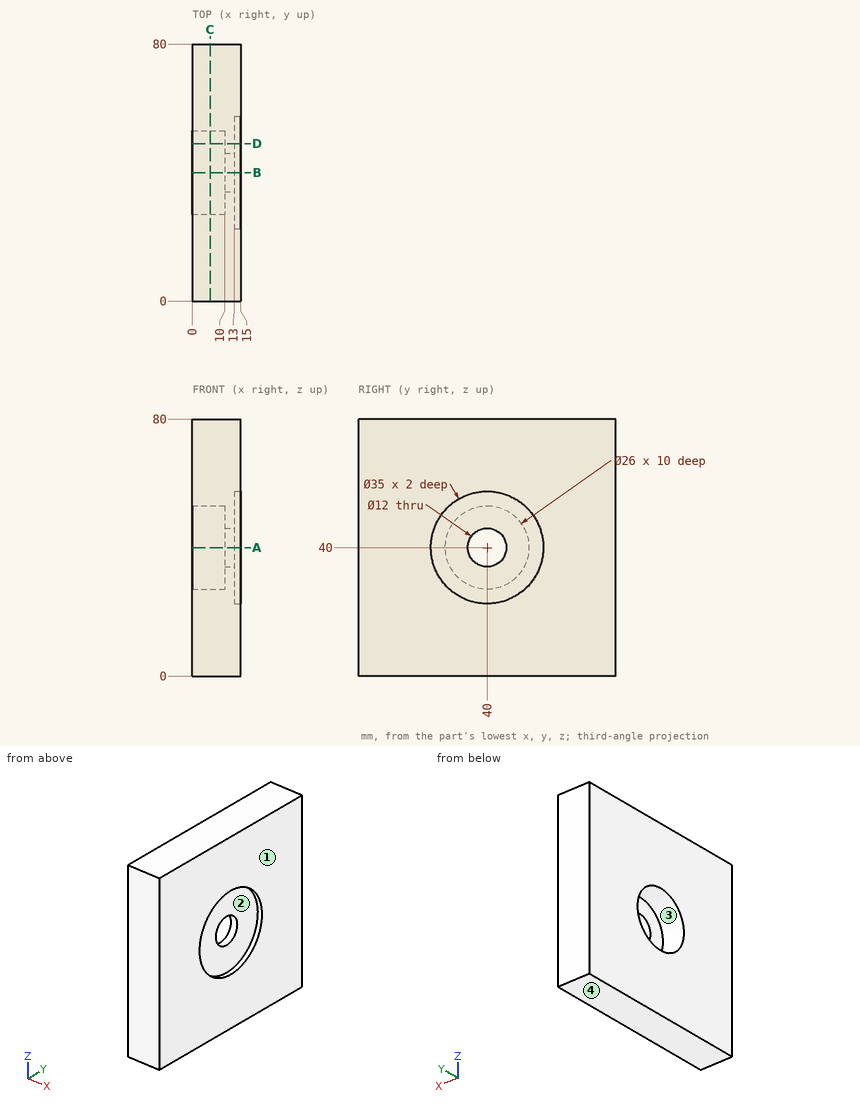
Check sheet for the drawn part. Datum: minimum x, y, z corner. Units: mm. Round coordinates to 2 decimals unless told otherwise and drop trailing zeros. Order: outer loops, then holes, each group sorted by start corner. A loop starts at its lowest first (then second) coordinate and runs counter-clockwise, first axis right, second up. Notation, with made-up numbers: M 17,69 L 26,69 A25 cw 26,100 Z; hole C -17,-21 d8. An arc over 180 degrees is marked long. Answer in a Markdown table with one row per item.
(1) Section check C-C on x = 5.5. Record the boundary of the cut face in (y, z).
Findings:
| item | result |
|---|---|
| outline | M 0,0 L 80,0 L 80,80 L 0,80 Z; hole C 40,40 d26 |
(2) Section check A-A on z = 40. Record the boundary of the cut face in (x, y), plus the area to 3 significant figures.
Findings:
| item | result |
|---|---|
| outline | M 0,0 L 15,0 L 15,22.5 L 13,22.5 L 13,34 L 10,34 L 10,27 L 0,27 Z; M 0,53 L 10,53 L 10,46 L 13,46 L 13,57.5 L 15,57.5 L 15,80 L 0,80 Z |
| area | 834 mm^2 |
(3) Section check D-D on y = 49. Record the boundary of the cut face in (x, z), plus the area to 3 significant figures.
Findings:
| item | result |
|---|---|
| outline | M 0,0 L 15,0 L 15,24.99 L 13,24.99 L 13,55.01 L 15,55.01 L 15,80 L 0,80 L 0,49.38 L 10,49.38 L 10,30.62 L 0,30.62 Z |
| area | 952 mm^2 |
(4) Gauge pin test, flat ends, axial feed: pin 1 (11 mm diameter, centred on y = 40, z = 40, fed in from +X); pin 2 (6 mm diameter, centred on x = 7, y = 68.5, fed in from -Z); pin 3 (17.5 mm diameter, centred on y = 47, z = 36, fed in from +X); pin 4 (8 mm diameter, centred on y = 43.5, z = 43.5, fed in from -X). Record the tip position at first contact, or that the pin passes through.
Findings:
| item | result |
|---|---|
| pin 1 | passes through |
| pin 2 | stops at z = 0 |
| pin 3 | stops at x = 13 |
| pin 4 | stops at x = 10 |
(5) Draft check along Z on the marked faces 1, 2, 3 and 4. Enter one of: +Z half, -Z half, draft (parallel to the pull), parting line (faces both ways), or undercut.
Findings:
| item | result |
|---|---|
| face 1 | draft |
| face 2 | undercut |
| face 3 | undercut |
| face 4 | -Z half |
(6) Material ranges on line 1 along Y through (x, z) = (4, 40); line 2 along Y through (x, z) = (11.7, 40); line 3 along Z through (x, y) = (8.25, 37), recorded low to high. Write a range as from..to.
Findings:
| item | result |
|---|---|
| line 1 | y = 0..27, 53..80 |
| line 2 | y = 0..34, 46..80 |
| line 3 | z = 0..27.35, 52.65..80 |
